Part model, mm, in its own coordinate system. Face numbers are marked on the shaded views. A direction names the side the tool comes from. Give positions to 0.01 mm unless a question says otherwise; leave off trailing zeros. Write each loop counter-clockwise with the first axis right and the second up, starting at its lowest first coordinate (ties: lowest second). Pieces come first, ordered by that corner, then holes. Notation, with made-up numbers: (-2.5, -4) - (42.5, -4) arc R21 ccw to (42.5, 12) - close; hole circle Ø7 at (-30.75, 82.5). An arc over 180 degrees is marked (long way). Answer in a Markdown table with one row per item. Add a question column.
1. Band-saw the part on D-D on x = 0. Write the cut outline in (y, z), plus the area to 3 significant figures.
2. Band-saw the part on B-B on y = 0. Write the cut outline in (x, z).
3. Band-saw the part on C-C on z = 4.75. Write the cut outline in (x, y).
4. Band-saw the part on A-A on z = 1. Write the cut outline in (x, y).
5. Which spindle directions (+Z, -Z, +X, -X, +Y, -Y) get a long thin tool onto all of the face, cutting with end or side? Do the marked faces 1, 2 and 3. Say none if no direction does.
6. Pull direction Y, two halves, no side cores. Call the marked faces 4, 5 and 6: released by +Y, released by -Y, zero draft, split by the parting line, or undercut.
7. Drop flat-ended pins along their axis: pin 1 Ø2.5 at (x, z) = (-1, 3) entering from +Y; pin 2 Ø3 at (x, z) = (-7, 4.5) entering from -Y; pin 3 Ø3.5 at (y, z) = (-25, 3) entering from -X. Give the stop position or say it passes through.
8. Probe line 1 along Z through (x, y) = (-7, 9); line 2 along Y through (x, z) = (-6, 4.75); line 3 along Y through (x, z) = (0, 12.6). List the from-to ranges inside material, lowest first.
```python
from build123d import *

# Parameters (mm, degrees)
F3_DEPTH         = 17.5
F5_DEPTH         = 12.801
F5_COPIES2_COUNT = 2
F6_W             = 22
F6_H             = 3
F7_DEPTH         = 12.801


# Not quite as in the source:
# - a pattern or mirror of a feature is missing from the dataset's text; its kind, count and spacing are read off the source's solid


with BuildPart() as f1:
    # F0 (on Front) → F1 (revolve)
    with BuildSketch(Plane.XZ):
        Polygon((-15, 0), (0, 0), (0, 12.4), (-17.75, 12.4), (-17.75, 12.8), (-18.25, 12.8), (-20, 11.5), (-20, 11.1382370815), (-22, 10.5), (-22, 2), (-19, 2), align=None)
    revolve(axis=Axis((0, 0, 3.4052523688), (0, 0, -1)))

    # F2 (on Right) → F3 (join, symmetric)
    with BuildSketch(Plane.YZ):
        with BuildLine():
            Line((23, 0), (25, 0))
            Line((25, 0), (27, 2))
            Line((27, 2), (20.8964254043, 8.9755138236))
            ThreePointArc((20.8964254043, 8.9755138236), (19.8783441675, 9.7318987418), (18.6386953202, 10))
            Line((18.6386953202, 10), (13, 10))
            Line((13, 10), (13, 4))
            Line((13, 4), (23, 0))
        make_face()
    f3 = extrude(amount=F3_DEPTH, both=True)

    # F3_copies: F3 across plane
    add(f3.mirror(Plane(origin=(0, 0, 0), x_dir=(0, 0, -1), z_dir=(0, -1, 0))))

    # F4 (on Top) → F5 (cut, through all)
    with BuildSketch(Plane.XY):
        Polygon((-17.5, 27), (-17.5, 13.332291626), (-15.5, 27), align=None)
    f5 = extrude(amount=F5_DEPTH, mode=Mode.SUBTRACT)

    # F5_copies: F5 across plane
    add(f5.mirror(Plane(origin=(0, 0, 0), x_dir=(0, 0, 1), z_dir=(1, 0, 0))), mode=Mode.SUBTRACT)

    # F5_copies1: F5 across plane
    add(f5.mirror(Plane(origin=(0, 0, 0), x_dir=(0, 0, -1), z_dir=(0, -1, 0))), mode=Mode.SUBTRACT)

    # F5_copies2: F5 ×2 about axis
    f5_copies2_axis = Axis((0, 0, 0), (0, 0, 1))
    for i in range(1, F5_COPIES2_COUNT):
        add(f5.rotate(f5_copies2_axis, i * 360 / F5_COPIES2_COUNT), mode=Mode.SUBTRACT)

    # F6 (on Top) → F7 (cut, through all)
    with BuildSketch(Plane.XY):
        with Locations((0, 25.5)):
            Rectangle(F6_W, F6_H)
    f7 = extrude(amount=F7_DEPTH, mode=Mode.SUBTRACT)

    # F7_copies: F7 across plane
    add(f7.mirror(Plane(origin=(0, 0, 0), x_dir=(0, 0, -1), z_dir=(0, -1, 0))), mode=Mode.SUBTRACT)


solid = f1.part
```
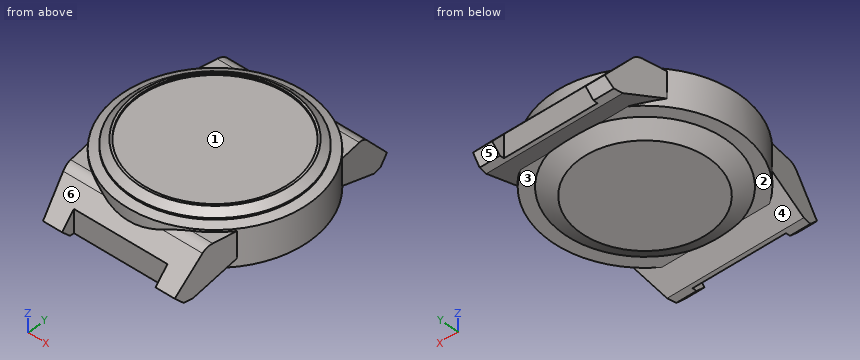
Values:
| question | item | result |
|---|---|---|
| 1 | outline | (-24, 0) - (-23, 0) - (-18.56, 1.78) - (-15, 0) - (15, 0) - (18.56, 1.78) - (23, 0) - (24, 0) - (24, 5.43) - (22, 7.71) - (22, 10.5) - (20, 11.14) - (20, 11.5) - (18.25, 12.8) - (17.75, 12.8) - (17.75, 12.4) - (-17.75, 12.4) - (-17.75, 12.8) - (-18.25, 12.8) - (-20, 11.5) - (-20, 11.14) - (-22, 10.5) - (-22, 7.71) - (-24, 5.43) - close |
| 1 | area | 551 mm² |
| 2 | outline | (-22, 2) - (-19, 2) - (-15, 0) - (15, 0) - (19, 2) - (22, 2) - (22, 10.5) - (20, 11.14) - (20, 11.5) - (18.25, 12.8) - (17.75, 12.8) - (17.75, 12.4) - (-17.75, 12.4) - (-17.75, 12.8) - (-18.25, 12.8) - (-20, 11.5) - (-20, 11.14) - (-22, 10.5) - close |
| 3 | outline | (-17.5, -13.33) - (-15.85, -24.59) - (-11, -24.59) - (-11, -24) - (11, -24) - (11, -24.59) - (15.85, -24.59) - (17.5, -13.33) arc R22 ccw to (17.5, 13.33) - (15.85, 24.59) - (11, 24.59) - (11, 24) - (-11, 24) - (-11, 24.59) - (-15.85, 24.59) - (-17.5, 13.33) arc R22 ccw to start |
| 4 | outline | circle Ø34 at (0, 0); (-16.45, -20.5) - (-15.65, -26) - (-11, -26) - (-11, -24) - (11, -24) - (11, -26) - (15.65, -26) - (16.45, -20.5) - close; (-16.45, 20.5) - (16.45, 20.5) - (15.65, 26) - (11, 26) - (11, 24) - (-11, 24) - (-11, 26) - (-15.65, 26) - close |
| 5 | face 1 | +Z |
| 5 | face 2 | -Z, -X |
| 5 | face 3 | -Z, +X |
| 6 | face 4 | undercut |
| 6 | face 5 | released by +Y |
| 6 | face 6 | released by -Y |
| 7 | pin 1 | stops at y = 24 |
| 7 | pin 2 | stops at y = -24 |
| 7 | pin 3 | stops at x = -16.05 |
| 8 | line 1 | z = 0 to 12.4 |
| 8 | line 2 | y = -24 to 24 |
| 8 | line 3 | y = -18.52 to -17.75, 17.75 to 18.52 |
